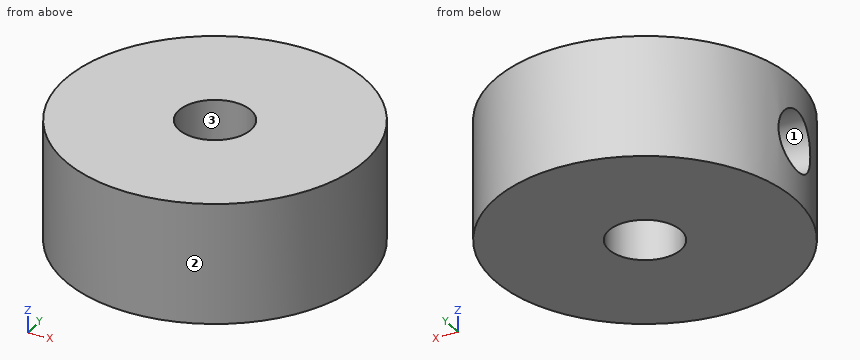
```python
from build123d import *

# Parameters (mm, degrees)
F0_R     = 9.525
F1_DEPTH = 7.62
F2_R     = 2.286
F3_DEPTH = 25.4
F4_R     = 1.905
F5_DEPTH = 25.4


with BuildPart() as f1:
    # F0 (on Top) → F1 (new body)
    with BuildSketch(Plane.XY):
        Circle(F0_R)
    extrude(amount=F1_DEPTH)

    # F2 (on face) → F3 (cut)
    with BuildSketch(Plane.XY.offset(7.62)):
        Circle(F2_R)
    extrude(amount=-F3_DEPTH, mode=Mode.SUBTRACT)

    # F4 (on Right) → F5 (cut)
    with BuildSketch(Plane.YZ):
        with Locations((0, 3.81)):
            Circle(F4_R)
    extrude(amount=-F5_DEPTH, mode=Mode.SUBTRACT)


solid = f1.part
```
Could you check a few things on this model? Use its own coordinates, in mm. Face numbers are marked on the shaded views. Round coordinates to 2 decimals unless told otherwise and drop trailing zeros. Loops run counter-clockwise (first coordinate to the right, second up) from the corner with the lowest first, then second, coordinate; pieces in that order, holes last. Notation, with made-up numbers: (-10, -37.5) - (6, -37.5) arc R16 cw to (6, -31.5) - close; hole circle Ø10 at (-19.75, 57.25). An arc over 180 degrees is marked (long way). Answer as CSV lines item,"result".
1. I want a section at D-D on z = 1.5. List the corners of the cut face in (x, y) for me (3 decimals).
Filled in:
outline,"circle Ø19.05 at (0, 0); hole circle Ø4.572 at (0, 0)"
2. We'd pull the mould along X, two halves only. Please class the marked faces 1, 2 and 3: +X half, -X half, draft (parallel to the pull), parting line (faces both ways), or undercut.
Filled in:
face 1,"draft"
face 2,"parting line"
face 3,"undercut"
3. I want a section at C-C on x = -5. List the corners of the cut face in (y, z) for me (3 decimals).
Filled in:
outline,"(-8.107, 0) - (8.107, 0) - (8.107, 7.62) - (-8.107, 7.62) - close; hole circle Ø3.81 at (0, 3.81)"
4. I want a section at A-A on y = 0. List the corners of the cut face in (x, z) for me (3 decimals).
Filled in:
outline,"(-9.525, 0) - (-2.286, 0) - (-2.286, 1.905) - (-9.525, 1.905) - close; (-9.525, 5.715) - (-2.286, 5.715) - (-2.286, 7.62) - (-9.525, 7.62) - close; (2.286, 0) - (9.525, 0) - (9.525, 7.62) - (2.286, 7.62) - close"
5. For pin 1 Ø3.5 at (y, z) = (0, 3.81) entering from -X; pin 2 Ø1.5 at (y, z) = (-0.5, 4.5) entering from -X; pin 3 Ø4 at (y, z) = (4, 6.5) entering from +X, each with a flat end and sliding along its axis, tell me the tip position at first contact or that it passes through.
Filled in:
pin 1,"stops at x = 1.47"
pin 2,"stops at x = 1.91"
pin 3,"stops at x = 9.31"
6. Please list where these lines run through material, in increasing order: line 1 along X through (y, z) = (0, 6) (3 decimals); line 2 along Y through (x, z) = (-4, 3.81) (3 decimals). Write a range as [from, to].
Filled in:
line 1,"x = [-9.525, -2.286], [2.286, 9.525]"
line 2,"y = [-8.644, -1.905], [1.905, 8.644]"
7. I want a section at B-B on x = 0. List the corners of the cut face in (y, z) for me (3 decimals).
Filled in:
outline,"(-9.525, 0) - (-2.286, 0) - (-2.286, 7.62) - (-9.525, 7.62) - close; (2.286, 0) - (9.525, 0) - (9.525, 7.62) - (2.286, 7.62) - close"
